The model under review builds one solid part; all positions refer to its coordinate system, in mm. A direction names the side the tool comes from. Round coordinates to 2 decimals unless told otherwise and drop trailing zeros. Order: outer loops, then holes, each group sorted by start corner. A loop starts at its lowest first (then second) coordinate and runs counter-clockwise, first axis right, second up.
1) Consider section D-D (x = 38.5). Give the boundary of the cut face in (y, z).
2) Consider section C-C (z = 1.6). Give the number of separate pieces and of enclosed holes in the cut face, then the cut area to 3 significant figures.
3) Consider section A-A (x = 65.5). Give the boundary of the cut face in (y, z).
4) Consider section B-B (y = 0). Give the boundary of the cut face in (x, z), then the cut area to 3 significant figures.
5) To check wall thickness, follow L1, parallel to Y at x = -75, z = 2.05; L2, parallel to Y at x = 27, z = 0.5; L3, parallel to X at y = -2.5, z = 1.45. State the ranges of each line that lie inside material, in increasing order.
6) Mouldability with a two-part tool opening along Y and no side actions: class faces 1 (the face through (1, 0, 0)), 2 (the face through (-30, 0, 1)), 3 (the face through (-64, 20, 1)) as pulls with the +Y half, pulls with the -Y half, needs draft (parallel to the pull), parting line crosses it, or undercut.
7) Machinability: for faces 4 (the face through (100, 0, 1)), 5 (the face through (26, -15, 1)), 6 (the face through (29, 15, 1)), 7 (the face through (20, -5, 1)), which of the approach directions +Z, -Z, +X, -X, +Y, -Y give a long, thin tool a straight path to every point of the face, cutting with its end or side? Answer none if there is none.
8) Clearance check with flat-ended pins moving along their axes: P1, Ø0.9, axis at x = 59.5, z = 1, coming from the -Y side; P2, Ø5, axis at x = -75, y = 0, coming from the -Z side; P3, Ø1, axis at y = -8, z = 0.5, coming from the -X side; P4, Ø5, axis at x = -56.5, y = -14, coming from the -Z side. State where each tip first meets the part, or that it passes through.
from build123d import *

# Parameters (mm, degrees)
SKETCH1_R           = 4
BOSS_EXTRUDE1_DEPTH = 3
FILLET1_R           = 5
SKETCH2_W           = 20
SKETCH2_H           = 10
CUT_EXTRUDE1_DEPTH  = 3
FILLET2_R           = 2
CUT_EXTRUDE3_DEPTH  = 3
FILLET4_R           = 5


with BuildPart() as part:
    # Sketch1 → Boss-Extrude1 (new body)
    with BuildSketch(Plane.XY):
        Polygon((-50, -25), (-50, -15), (100, -15), (100, 15), (-50, 15), (-50, 25), (-100, 25), (-100, -25), align=None)
        with Locations((-75, 0)):
            Circle(SKETCH1_R, mode=Mode.SUBTRACT)
    extrude(amount=BOSS_EXTRUDE1_DEPTH)

    # Fillet1
    fillet1_edges = [part.edges().sort_by_distance(p)[0] for p in [
        (-50, -15, 1.5),
        (-50, 15, 1.5),
    ]]
    fillet(fillet1_edges, radius=FILLET1_R)
    fillet1_2_edges = [part.edges().sort_by_distance(p)[0] for p in [
        (-50, -25, 1.5),
        (-50, 25, 1.5),
    ]]
    fillet(fillet1_2_edges, radius=FILLET1_R - 0.0001)  # a hair under: the kernel refuses the full size

    # Sketch2 → Cut-Extrude1 (cut)
    with BuildSketch(Plane(origin=(0, 0, 0), x_dir=(-1, 0, 0), z_dir=(0, 0, -1))):
        with Locations((20, 0)):
            Rectangle(SKETCH2_W, SKETCH2_H)
        with Locations((-20, 0)):
            Rectangle(SKETCH2_W, SKETCH2_H)
        with Locations((-60, 0)):
            Rectangle(SKETCH2_W, SKETCH2_H)
    extrude(amount=-CUT_EXTRUDE1_DEPTH, mode=Mode.SUBTRACT)

    # Fillet2
    fillet2_edges = [part.edges().sort_by_distance(p)[0] for p in [
        (-30, -5, 1.5),
        (-10, -5, 1.5),
        (-10, 5, 1.5),
        (-30, 5, 1.5),
        (30, 5, 1.5),
        (10, 5, 1.5),
        (10, -5, 1.5),
        (30, -5, 1.5),
        (70, 5, 1.5),
        (50, 5, 1.5),
        (50, -5, 1.5),
        (70, -5, 1.5),
    ]]
    fillet(fillet2_edges, radius=FILLET2_R)

    # Sketch3 → Cut-Extrude3 (cut)
    with BuildSketch(Plane(origin=(0, 0, 0), x_dir=(-1, 0, 0), z_dir=(0, 0, -1))):
        with BuildLine():
            ThreePointArc((75, -20), (95, 0), (75, 20))
            Line((75, 20), (50, 20))
            ThreePointArc((50, 20), (51.464466094, 23.535533906), (55, 25))
            Line((55, 25), (100, 25))
            Line((100, 25), (100, -25))
            Line((100, -25), (55, -25))
            ThreePointArc((55, -25), (51.464466094, -23.535533906), (50, -20))
            Line((50, -20), (75, -20))
        make_face()
    extrude(amount=-CUT_EXTRUDE3_DEPTH, mode=Mode.SUBTRACT)


with BuildPart() as cut_extrude3_kept_piece:
    # of the separate pieces the step leaves, the one the design keeps (cut_extrude3_pieces_kept)
    add(part.part.solids().sort_by_distance((-50, -20, 0))[0])

    # Fillet4
    fillet4_edges = [cut_extrude3_kept_piece.edges().sort_by_distance(p)[0] for p in [
        (-50, -20, 1.5),
        (-50, 20, 1.5),
    ]]
    fillet(fillet4_edges, radius=FILLET4_R)


solid = cut_extrude3_kept_piece.part
Answer below:
1. outline: (-15, 0) - (15, 0) - (15, 3) - (-15, 3) - close
2. separate pieces: 1
2. enclosed holes: 4
2. area: 5,500 mm2
3. outline: (-15, 0) - (-5, 0) - (-5, 3) - (-15, 3) - close; (5, 0) - (15, 0) - (15, 3) - (5, 3) - close
4. outline: (-95, 0) - (-79, 0) - (-79, 3) - (-95, 3) - close; (-71, 0) - (-30, 0) - (-30, 3) - (-71, 3) - close; (-10, 0) - (10, 0) - (10, 3) - (-10, 3) - close; (30, 0) - (50, 0) - (50, 3) - (30, 3) - close; (70, 0) - (100, 0) - (100, 3) - (70, 3) - close
4. area: 381 mm2
5. L1: y = -20 to -4, 4 to 20
5. L2: y = -15 to -5, 5 to 15
5. L3: x = -94.84 to -78.12, -71.88 to -30, -10 to 10, 30 to 50, 70 to 100
6. face 1: needs draft
6. face 2: undercut
6. face 3: pulls with the +Y half
7. face 4: +Z, -Z, +X, +Y, -Y
7. face 5: +Z, -Z, +X, -Y
7. face 6: +Z, -Z, +X, +Y
7. face 7: +Z, -Z
8. P1: stops at y = -15
8. P2: passes through
8. P3: stops at x = -93.54
8. P4: stops at z = 0
